Here's how the part is built. I have some questions about the finished solid (model axes, mm). Face numbers are marked on the shaded views. A direction names the side the tool comes from. Coordinates: 2 decimals unless noted, no trailing zeros. Write each loop counter-clockwise with the first axis right and the second up, starting at its lowest first coordinate (ties: lowest second). Pieces come first, ordered by that corner, then holes.
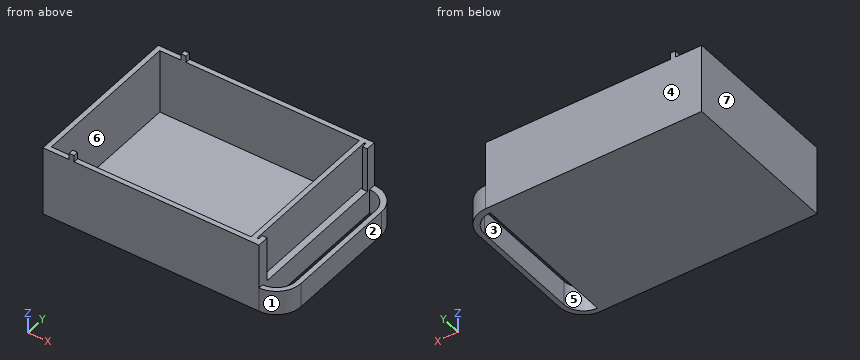
Autodesk Inventor part; units mm, degrees
ref_plane "YZ Plane" through (0, 0, 0) normal (1, 0, 0) x (0, 1, 0)
ref_plane "XZ Plane" through (0, 0, 0) normal (0, 1, 0) x (-1, 0, 0)
ref_plane "XY Plane" through (0, 0, 0) normal (0, 0, 1) x (1, 0, 0)
sketch "Sketch1" plane through (0, 0, 0) normal (0, 0, 1) x (1, 0, 0)
  line L0 (0, 0) -> (132, 0)
  line L1 (0, 0) -> (132, 0)
  line L2 (0, 0) -> (132, 0)
  line L3 (132, 0) -> (132, 99)
  line L4 (132, 99) -> (0, 99)
  line L5 (0, 99) -> (0, 0)
  dimension "d12" = 132
  dimension "d13" = 99
extrude "Extrusion2" add sketch "Sketch1" along normal blind 3
sketch "Sketch2" plane through (0, 0, 3) normal (0, 0, 1) x (1, 0, 0)
  line L0 (3, 96) -> (125, 96)
  line L1 (125, 96) -> (125, 3)
  line L2 (125, 3) -> (3, 3)
  line L3 (3, 3) -> (3, 96)
  line L4 (132, 99) -> (0, 99)
  line L5 (0, 0) -> (132, 0)
  line L6 (0, 99) -> (0, 0)
  line L7 (132, 0) -> (132, 99)
  dimension "d16" = 3
  dimension "d17" = 3
  dimension "d18" = 3
  dimension "d21" = 7
extrude "Extrusion3" add sketch "Sketch2" along normal blind 12
sketch "Sketch3" plane through (0, 0, 0) normal (0, 0, -1) x (-1, 0, 0)
  point P0 (0, 0)
sketch "Sketch4" plane through (0, 0, 0) normal (0, 0, -1) x (-1, 0, 0)
  line L0 (-132, 99) -> (0, 99)
  line L1 (-132, 99) -> (-132, 84)
  line L2 (-132, 0) -> (-132, 99)
  line L3 (-132, 0) -> (-132, 15)
  arc A0 (-147, 15) -> (-132, 0) centre (-132, 15) ccw
  line L4 (-132, 15) -> (-147, 15) construction
  line L5 (-132, 15) -> (-132, 0) construction
  arc A1 (-132, 99) -> (-147, 84) centre (-132, 84) ccw
  line L6 (-132, 84) -> (-147, 84) construction
  line L7 (-132, 84) -> (-132, 99) construction
  line L8 (-147, 84) -> (-147, 15)
  point P0 (0, 0)
  dimension "d24" = 15
  dimension "d25" = 15
  dimension "d26" = 90
  dimension "d27" = 90
extrude "Extrusion4" add sketch "Sketch4" against normal blind 15
sketch "Sketch5" plane through (0, 0, 0) normal (0, 0, -1) x (-1, 0, 0)
  line L0 (-132, 99) -> (0, 99)
  line L1 (0, 0) -> (-132, 0)
  arc A0 (-132, 95) -> (-144, 83) centre (-132, 83) ccw
  arc A1 (-144, 15) -> (-132, 3) centre (-132, 15) ccw
  line L2 (-144, 83) -> (-144, 15)
  line L3 (-132, 95) -> (-132, 3)
  dimension "d35" = 3
  dimension "d36" = 92
  dimension "d37" = 3
extrude "Extrusion5" cut sketch "Sketch5" against normal through all
sketch "Sketch6" plane through (0, 0, 15) normal (0, 0, 1) x (1, 0, 0)
  line L0 (132, 99) -> (0, 99)
  arc A0 (147, 84) -> (132, 99) centre (132, 84) ccw
  line L1 (0, 99) -> (132, 99)
  line L2 (132, 99) -> (132, 93)
  line L3 (132, 3) -> (132, 95)
  line L4 (132, 93) -> (129, 93)
  line L5 (129, 93) -> (129, 96)
  line L6 (129, 96) -> (128, 96)
  line L7 (128, 96) -> (128, 4)
  line L8 (125, 96) -> (125, 3)
  line L9 (128, 4) -> (129, 4)
  line L10 (129, 4) -> (129, 7)
  line L11 (129, 7) -> (132, 7)
  line L12 (132, 7) -> (132, 0)
  line L13 (0, 0) -> (132, 0)
  line L14 (132, 0) -> (0, 0)
  line L15 (0, 99) -> (0, 0)
  line L16 (0, 0) -> (0, 99)
  line L17 (3, 96) -> (125, 96)
  line L18 (3, 96) -> (125, 96)
  line L19 (125, 96) -> (125, 3)
  line L20 (125, 3) -> (3, 3)
  line L21 (3, 3) -> (3, 96)
  dimension "d40" = 6
  dimension "d41" = 3
  dimension "d42" = 3
  dimension "d43" = 1
  dimension "d44" = 3
  dimension "d45" = 3
extrude "Extrusion6" add sketch "Sketch6" along normal blind 27.5 contours L2 L4 L5 L6 L7 L9 L10 L11 L3 L12 L13 L15 L0
sketch "Sketch7" plane through (0, 0, 42.5) normal (0, 0, 1) x (1, 0, 0)
  line L0 (0, 99) -> (0, 0)
  line L1 (0, 0) -> (16, 0)
  line L2 (0, 0) -> (132, 0)
  line L3 (3, 3) -> (125, 3)
  line L4 (16, 0) -> (19, 0)
  line L5 (19, 0) -> (19, 3)
  line L6 (19, 3) -> (16, 3)
  line L7 (16, 3) -> (16, 0)
  line L8 (0, 99) -> (16, 99)
  line L9 (132, 99) -> (0, 99)
  line L10 (125, 96) -> (3, 96)
  line L11 (16, 99) -> (19, 99)
  line L12 (19, 99) -> (19, 96)
  line L13 (19, 96) -> (16, 96)
  line L14 (16, 96) -> (16, 99)
  dimension "d48" = 16
  dimension "d49" = 3
  dimension "d50" = 16
  dimension "d51" = 3
extrude "Extrusion7" add sketch "Sketch7" along normal blind 4
sketch "Sketch10" plane through (0, 0, 0) normal (0, -1, 0) x (1, 0, 0)
  line L0 (132, 42.5) -> (19, 42.5)
  line L1 (19, 42.5) -> (22, 42.5)
  line L2 (22, 3) -> (22, 0)
  line L3 (0, 0) -> (132, 0)
  line L4 (0, 0) -> (0, 22)
  line L5 (0, 0) -> (0, 42.5)
  line L6 (0, 22) -> (3, 22)
  arc A0 (0, 22) -> (22, 0) centre (22, 22) ccw
  line L7 (125, 3) -> (3, 3)
  arc A1 (3, 22) -> (22, 3) centre (22, 22) ccw
  line L8 (19, 3.2383) -> (19, 3)
  line L9 (19, 0.2055) -> (19, 0)
  dimension "d70" = 3
  dimension "d73" = 22
  dimension "d74" = 3
  dimension "d75" = 3
  dimension "d76" = 19
equation "\"d16\" = d17"
equation "\"d18\" = d17"
equation "\"d25\" = d24"
equation "\"d35\" = d17"
equation "\"d37\" = d17"
equation "\"d41\" = d17"
equation "\"d42\" = d17"
equation "\"d44\" = d17"
equation "\"d45\" = d17"
equation "\"d49\" = d17"
equation "\"d51\" = d17"
equation "\"d70\" = d17"
equation "\"d74\" = d17"
equation "\"d75\" = d17"
properties part number "boxMVer1"
1. Thinking about a two-plate mould opening in Y: for the marked faces 1, 2, 3 and 4, which applies, pulls with the +Y half, pulls with the -Y half, needs draft (parallel to the pull), parting line crosses it, or undercut?
2. For pin 1 Ø4.5 at (x, y) = (129.5, 67.5) entering from +Z; pin 2 Ø1.5 at (x, y) = (56, 29) entering from +Z; pin 3 Ø1.5 at (y, z) = (1, 45) entering from -X, each with a flat end and sliding along its axis, tell me the tip position at first contact or that it passes through.
3. I want a section at B-B (z = 12). List the corners of the cut face in (x, y) for me.
4. I want a section at D-D (z = 28). List the corners of the cut face in (x, y) for me, then the cut area to 3 significant figures.
5. If I drill on line 1 (X direction, y = 70, z = 6); line 2 (X direction, y = 6.5, z = 30); line 3 (Y direction, x = 36, z = 11), over which ranges is the centre line in solid material (lowest first)?
6. On a 3-axis mill with a long thin cutter (end or side, diameter ignored), from which of +Z, -Z, +X, -X, +Y, -Y can I reach the whole of each face in a straight line? I mean the marked faces 5, 6 and 7. Say none if no direction works.
7. I want a section at C-C (x = 43.5). List the corners of the cut face in (y, z) for me, then the cut area to 3 significant figures.
8. I want a section at A-A (y = 17). List the corners of the cut face in (x, z) for me, then the cut area to 3 significant figures.
Response values:
1. face 1: pulls with the -Y half
1. face 2: needs draft
1. face 3: undercut
1. face 4: pulls with the +Y half
2. pin 1: stops at z = 42.5
2. pin 2: stops at z = 3
2. pin 3: stops at x = 16
3. outline: (0, 0) - (132, 0) arc R15 ccw to (147, 15) - (147, 84) arc R15 ccw to (132, 99) - (0, 99) - close; hole (3, 3) - (125, 3) - (125, 96) - (3, 96) - close; hole (132, 3) arc R12 ccw to (144, 15) - (144, 83) arc R12 ccw to (132, 95) - close
4. outline: (0, 0) - (132, 0) - (132, 7) - (129, 7) - (129, 4) - (128, 4) - (128, 96) - (129, 96) - (129, 93) - (132, 93) - (132, 99) - (0, 99) - close; hole (3, 3) - (125, 3) - (125, 96) - (3, 96) - close
4. area: 1,370 mm2
5. line 1: x = 0 to 3, 125 to 132, 144 to 147
5. line 2: x = 0 to 3, 125 to 128, 129 to 132
5. line 3: y = 0 to 3, 96 to 99
6. face 5: +Z, -Z
6. face 6: +Z
6. face 7: +Z, -Z, -X, +Y, -Y
7. outline: (0, 0) - (99, 0) - (99, 42.5) - (96, 42.5) - (96, 3) - (3, 3) - (3, 42.5) - (0, 42.5) - close
7. area: 534 mm2
8. outline: (0, 0) - (132, 0) - (132, 15) - (128, 15) - (128, 42.5) - (125, 42.5) - (125, 3) - (3, 3) - (3, 42.5) - (0, 42.5) - close; (144, 0) - (147, 0) - (147, 15) - (144, 15) - close
8. area: 726 mm2
